```python
from build123d import *

# Parameters (mm, degrees)
F0_R     = 21
F2_DEPTH = 2.38125
F1_R     = 8.73125
F3_DEPTH = 13.49375
F4_R     = 2.38125
F5_DEPTH = 11.1125
F7_DEPTH = 2.38125
F8_DEPTH = 2.38125


with BuildPart() as f2:
    # F0 (on Top) → F2 (new body)
    with BuildSketch(Plane.XY):
        Circle(F0_R)
    extrude(amount=F2_DEPTH)

    # F1 (on face) → F3 (join)
    with BuildSketch(Plane.XY):
        Circle(F1_R)
    extrude(amount=F3_DEPTH)

    # F4 (on face) → F5 (cut)
    with BuildSketch(Plane.XY.offset(13.49375)):
        Circle(F4_R)
    extrude(amount=-F5_DEPTH, mode=Mode.SUBTRACT)

    # F6 (on face) → F7 (cut)
    with BuildSketch(Plane(origin=(0, 0, 0), x_dir=(1, 0, 0), z_dir=(0, 0, -1))):
        with BuildLine():
            ThreePointArc((0, 15.6), (1.555635, 16.244365), (2.2, 17.8))
            ThreePointArc((2.2, 17.8), (-1.555635, 19.355635), (0, 15.6))
        make_face()
    extrude(amount=-F7_DEPTH, mode=Mode.SUBTRACT)

    # F6 (on face) → F8 (cut)
    with BuildSketch(Plane(origin=(0, 0, 0), x_dir=(1, 0, 0), z_dir=(0, 0, -1))):
        with BuildLine():
            ThreePointArc((0, 15.6), (1.555635, 16.244365), (2.2, 17.8))
            ThreePointArc((2.2, 17.8), (-1.555635, 19.355635), (0, 15.6))
        make_face()
        with BuildLine():
            ThreePointArc((18.809169, 2.424734), (15.034562, 5.913945), (11.85226, 1.877214))
            ThreePointArc((11.85226, 1.877214), (15.583776, -1.064476), (18.809169, 2.424734))
        make_face()
        with BuildLine():
            ThreePointArc((17.615252, -8.9), (15.984654, -6.774963), (13.509996, -7.8))
            ThreePointArc((13.509996, -7.8), (14.84585, -11.025037), (17.615252, -8.9))
        make_face()
        with BuildLine():
            ThreePointArc((-13.215252, -8.9), (-13.290215, -8.330598), (-13.509996, -7.8))
            ThreePointArc((-13.509996, -7.8), (-17.540289, -9.469402), (-13.215252, -8.9))
        make_face()
    extrude(amount=-F8_DEPTH, mode=Mode.SUBTRACT)


solid = f2.part
```
Geometry: final body of the model. Coordinates: model frame, mm. A direction names the side the tool comes from. Give positions to 0.01 mm unless a question says otherwise; leave off trailing zeros. Order: outer loops, then holes, each group sorted by start corner. A loop starts at its lowest first (then second) coordinate and runs counter-clockwise, first axis right, second up. Notation, with made-up numbers: (85.5, 62.25) -> (137.5, 62.25) arc R15 ccw to (137.5, 70.25) -> close; hole circle Ø3 at (59.5, -35). An arc over 180 degrees is marked (long way). Write each question's results on one line, items separated by ' | '. Start each with the question number.
1) Section C-C (y = 0). Return loops of the section in (x, z).
2) Set-up query: faces 1 (the flat face through (2, -2, 13.494)), 2 (the flat face through (0, 0, 2.381)). Return all of +Z, -Z, +X, -X, +Y, -Y with unobstructed straight access to the full face (end or side cutting, diameter ignored); none if empty.
3) Section B-B (x = -16.5). Return loops of the section in (y, z).
4) Section A-A (z = 1.5). Return loops of the section in (x, y).
5) Draft query along X for faces 3 (the cylindrical face through (-6.93, -5.31, 7.86)), 4 (the flat face through (0, -9, 2.381)), 5 (the cylindrical face through (-1.89, -1.45, 8.02)). Return one class per face: pulls with the +X half, pulls with the -X half, needs draft (parallel to the pull), parting line crosses it, or undercut.
6) Section D-D (z = 4.5). Return loops of the section in (x, y), then the cut area to 3 significant figures.
7) First-contact query: pin 1 (12 mm diameter, centred on x = 16, y = -1, fed in from +Z); pin 2 (1.5 mm diameter, centred on x = 4.5, z = 6, fed in from +Y); pin 3 (4 mm diameter, centred on y = 0, z = 5, fed in from -X). Flat tips, straight axial feed; report the tip coordinate or a pass-through.
8) Line query: line 1 (X direction, y = 8.9, z = 1.95); line 2 (Y direction, x = 0, z = 10.5); line 3 (Y direction, x = 0, z = 0.65). Output: solid intervals per line, ascending. Write a range as from..to.
Calculated:
1) outline: (-21, 0) -> (12.79, 0) -> (12.79, 2.38) -> (8.73, 2.38) -> (8.73, 13.49) -> (2.38, 13.49) -> (2.38, 2.38) -> (-2.38, 2.38) -> (-2.38, 13.49) -> (-8.73, 13.49) -> (-8.73, 2.38) -> (-21, 2.38) -> close; (17.83, 0) -> (21, 0) -> (21, 2.38) -> (17.83, 2.38) -> close
2) face 1: +Z, +X, -X, +Y, -Y | face 2: +Z
3) outline: (-12.99, 0) -> (6.99, 0) -> (6.99, 2.38) -> (-12.99, 2.38) -> close; (10.81, 0) -> (12.99, 0) -> (12.99, 2.38) -> (10.81, 2.38) -> close
4) outline: circle Ø42 at (0, 0); hole (-13.51, 7.8) arc R2.2 ccw to (-13.22, 8.9) arc R2.2 ccw (long way) to start; hole circle Ø4.4 at (0, -17.8); hole circle Ø7 at (15.31, -2.42); hole circle Ø4.4 at (15.42, 8.9)
5) face 3: parting line crosses it | face 4: needs draft | face 5: undercut
6) outline: circle Ø17.46 at (0, 0); hole circle Ø4.76 at (0, 0) | area: 222 mm2
7) pin 1: z = 2.38 | pin 2: y = 7.88 | pin 3: x = -8.73
8) line 1: -19.02..-17.62, -13.22..13.22, 17.62..19.02 | line 2: -8.73..-2.38, 2.38..8.73 | line 3: -21..-20, -15.6..21
